Source: three-view drawing plus pictorial views. Frame: mm from the lowest corner of the part. A direction names the side the tool comes from. Coordinates: 2 decimals unless noted, no trailing zeros. Order: outer loops, then holes, each group sorted by start corner. A loop starts at its lowest first (then second) coordinate and runs counter-clockwise, first axis right, second up. Notation, with made-up numbers: (58.25, 87.25) -> (100.25, 87.25) arc R23 ccw to (100.25, 96.25) -> close; hole circle Ø10 at (-10.5, -18). An arc over 180 degrees is marked (long way). Use one line per item in the form item = value. Start each with the question number.
1) Access query for the marked faces 4, 5, 6 and 7. Directions: +Z, -Z, +X, -X, +Y, -Y. A direction counts if a zero-diameter tool reaches every point of the face in a straight line with its end or side. Return the directions, or none.
2) Section query D-D on x = 25. Output: boundary loops of the cut face in (y, z).
3) Pin query (flat end, axial travel): pin 1 (12 mm diameter, centred on x = 16.5, z = 13.5, fed in from +Y). Return the tip coordinate at first contact, or that it passes through.
4) Draft query along Y for the marked faces 1, 2 and 3. Return one class per face: pulls with the +Y half, pulls with the -Y half, needs draft (parallel to the pull), parting line crosses it, or undercut.
5) Section query C-C on z = 53. Output: boundary loops of the cut face in (x, y), then the cut area to 3 significant figures.
6) Section query B-B on z = 35.5. Output: boundary loops of the cut face in (x, y).
7) Section query A-A on y = 26. Output: boundary loops of the cut face in (x, z).
8) Ray query, line 1 along Z through (x, y) = (12, 10); line 2 along Y through (x, z) = (13, 37); line 3 along Z through (x, y) = (39, 7). Return the intervals inside material, ascending.
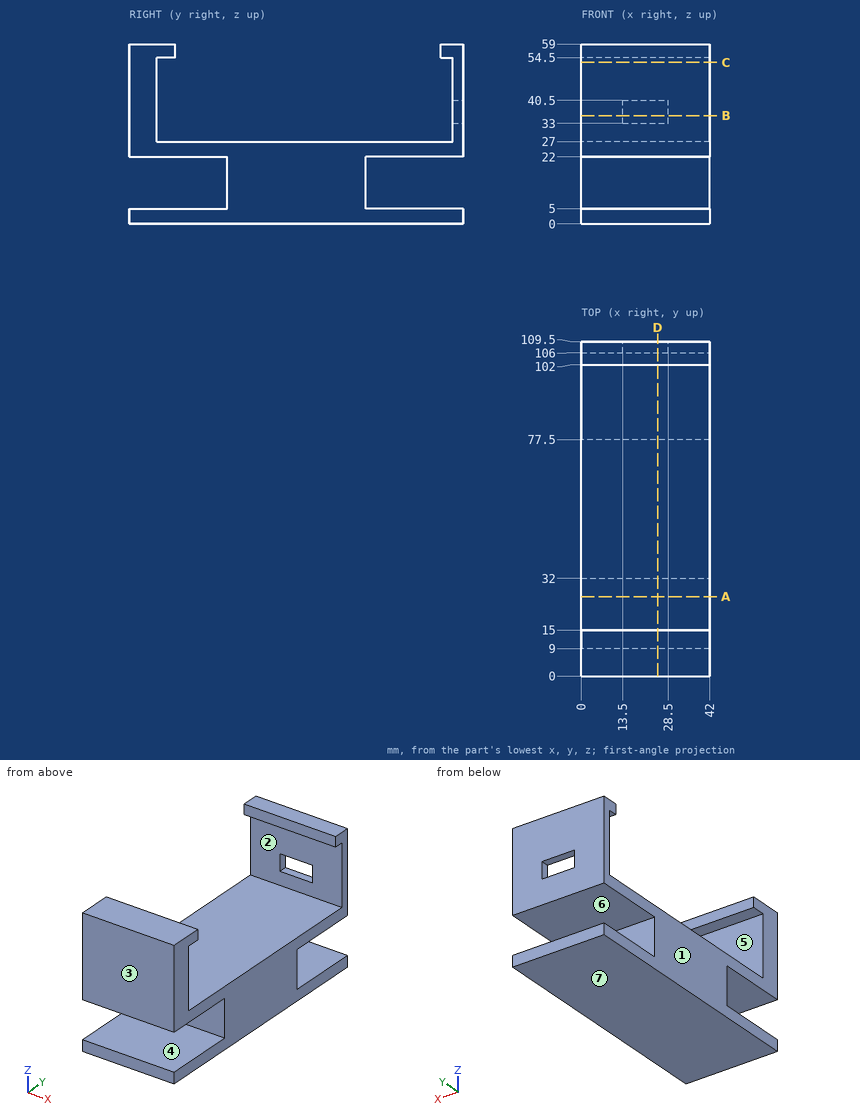
Answers below:
q1.face_4 = +X, -X, -Y
q1.face_5 = +X, -X
q1.face_6 = +X, -X, +Y
q1.face_7 = -Z, +X, -X, +Y, -Y
q2.outline = (0, 0) -> (109.5, 0) -> (109.5, 5) -> (77.5, 5) -> (77.5, 22) -> (109.5, 22) -> (109.5, 33) -> (106, 33) -> (106, 27) -> (9, 27) -> (9, 54.5) -> (15, 54.5) -> (15, 59) -> (0, 59) -> (0, 22) -> (32, 22) -> (32, 5) -> (0, 5) -> close; (102, 54.5) -> (106, 54.5) -> (106, 40.5) -> (109.5, 40.5) -> (109.5, 59) -> (102, 59) -> close
q3.pin_1 = 77.5
q4.face_1 = needs draft
q4.face_2 = undercut
q4.face_3 = pulls with the -Y half
q5.outline = (0, 0) -> (42, 0) -> (42, 9) -> (0, 9) -> close; (0, 106) -> (42, 106) -> (42, 109.5) -> (0, 109.5) -> close
q5.area = 525 mm^2
q6.outline = (0, 0) -> (42, 0) -> (42, 9) -> (0, 9) -> close; (0, 106) -> (13.5, 106) -> (13.5, 109.5) -> (0, 109.5) -> close; (28.5, 106) -> (42, 106) -> (42, 109.5) -> (28.5, 109.5) -> close
q7.outline = (0, 0) -> (42, 0) -> (42, 5) -> (0, 5) -> close; (0, 22) -> (42, 22) -> (42, 27) -> (0, 27) -> close
q8.line_1 = 0 to 5, 22 to 27, 54.5 to 59
q8.line_2 = 0 to 9, 106 to 109.5
q8.line_3 = 0 to 5, 22 to 59
